```python
from build123d import *

# Parameters (mm, degrees)
BOSS_EXTRUDE1_DEPTH = 25.4
SKETCH2_R           = 9.801448676
SKETCH2_R_2         = 7.071368029
BOSS_EXTRUDE2_DEPTH = 19
BOSS_EXTRUDE3_DEPTH = 3.175
SKETCH4_R           = 3.175
CUT_EXTRUDE1_DEPTH  = 3.175


with BuildPart() as part:
    # Sketch1 → Boss-Extrude1 (new body)
    with BuildSketch(Plane.XY):
        Polygon((-76.495819173, -3.422180745), (-20.941461675, -3.422180745), (-1.20885062, 35.305249012), (-7.464460479, 16.03438497), (-18.995819173, -6.597180745), (-76.495819173, -6.597180745), align=None)
    extrude(amount=BOSS_EXTRUDE1_DEPTH)

    # Sketch2 → Boss-Extrude2 (add)
    with BuildSketch(Plane(origin=(0, -3.422180745, 0), x_dir=(1, 0, 0), z_dir=(0, 1, 0))):
        with Locations((-76.495819173, -12.7)):
            Circle(SKETCH2_R)
        with Locations((-76.495819173, -12.7)):
            Circle(SKETCH2_R_2, mode=Mode.SUBTRACT)
    extrude(amount=-BOSS_EXTRUDE2_DEPTH)

    # Sketch3 → Boss-Extrude3 (add)
    with BuildSketch(Plane(origin=(0, -3.422180745, 0), x_dir=(1, 0, 0), z_dir=(0, 1, 0))):
        Polygon((-76.495819173, -25.4), (-76.495819173, 0), (-85.929582176, -10.040580563), (-85.929582176, -15.359419437), align=None)
        Polygon((-85.929582176, -15.359419437), (-85.929582176, -10.040580563), (-86.297267848, -12.7), align=None)
    extrude(amount=-BOSS_EXTRUDE3_DEPTH)

    # Sketch4 → Cut-Extrude1 (cut)
    with BuildSketch(Plane(origin=(-15.240970814, 7.765662505, 0), x_dir=(0, 0, 1), z_dir=(-0.891006524, 0.4539905, 0))):
        with Locations((12.7, 18.20840051)):
            Circle(SKETCH4_R)
    extrude(amount=-CUT_EXTRUDE1_DEPTH, mode=Mode.SUBTRACT)


solid = part.part
```
Check sheet for the modelled part. Datum: model origin and axes. Units: mm. A direction names the side the tool comes from. Give positions to 0.01 mm unless a question says otherwise; leave off trailing zeros. Write each loop counter-clockwise with the first axis right and the second up, starting at its lowest first coordinate (ties: lowest second). Pieces come first, ordered by that corner, then holes. Notation, with made-up numbers: (6, 79) - (39, 79) arc R18 cw to (39, 102) - close; hole circle Ø9 at (71.5, 75). An arc over 180 degrees is marked (long way). Answer as a JSON object with one key per item and string values. Group by question number.
1) Access from +Z, -Z, +X, -X, +Y, -Y to the whole of each face (thin tool, end or side, straight path). Record for faces 4 (the face through (-76, -6.597, 13)), 5 (the face through (-78.094, -4.987, 1.701)), 6 (the face through (-54, -3.422, 13)).
2) Sectioned sample at D-D (z = 16.75). Record the cut outline in (x, y), then the cut area to 3 significant figures.
3) Release check for a two-part mould opening along Z. For faces 1 (the face through (-36, -4, 0)), 2 (the face through (-7.49, 20.773, 12.012)), 3 (the face through (-86.288, -14.9, 12.269)) record: pulls with the +Z half, pulls with the -Z half, needs draft (parallel to the pull), parting line crosses it, or undercut.
4) Sectioned sample at A-A (z = 12.7). Record the cut outline in (x, y), then the cut area to 3 significant figures.
5) Sectioned sample at B-B (x = -24.5). Record the cut outline in (y, z), then the cut area to 3 significant figures.
6) Thickness scan on probe 1 along X at (y, z) = (-12, 12.7); probe 2 along Y at (x, z) = (-59.5, 17.5); probe 3 along X at (y, z) = (-18.5, 17.75). Record the ranges inside material, lowest first. Write a range as from..to.
7) Depth check by flat-ended pin: P1, Ø8, axis at x = -76, z = 12.5, coming from the +Y side; P2, Ø10, axis at x = -11.5, z = 6, coming from the +Y side; P3, Ø5, axis at y = -12, z = 9, coming from the -X side. Enter the tip coordinate at first touch or a pass-through.
8) Sectioned sample at C-C (z = 23.5). Record the cut outline in (x, y), then the cut area to 3 significant figures.
Geometry results:
{
 "1": {"face 4": "-Y", "face 5": "-Z, -X, +Y, -Y", "face 6": "+Z, -Z, -X, +Y"},
 "2": {"outline": "(-85.42, -22.42) - (-82.29, -22.42) - (-82.29, -6.6) - (-70.7, -6.6) - (-70.7, -22.42) - (-67.57, -22.42) - (-67.57, -6.6) - (-19, -6.6) - (-7.46, 16.03) - (-1.21, 35.31) - (-20.94, -3.42) - (-85.42, -3.42) - close", "area": "416 mm^2"},
 "3": {"face 1": "pulls with the -Z half", "face 2": "undercut", "face 3": "parting line crosses it"},
 "4": {"outline": "(-86.3, -22.42) - (-83.57, -22.42) - (-83.57, -6.6) - (-69.42, -6.6) - (-69.42, -22.42) - (-66.69, -22.42) - (-66.69, -6.6) - (-19, -6.6) - (-7.46, 16.03) - (-6.17, 20.02) - (-8.42, 21.16) - (-20.94, -3.42) - (-86.3, -3.42) - close; (-5.53, 26.82) - (-4.19, 26.13) - (-1.21, 35.31) - close", "area": "394 mm^2"},
 "5": {"outline": "(-6.6, 0) - (-3.42, 0) - (-3.42, 25.4) - (-6.6, 25.4) - close", "area": "80.6 mm^2"},
 "6": {"probe 1": "x = -86.3..-83.57, -69.42..-66.69", "probe 2": "y = -6.6..-3.42", "probe 3": "x = -84.9..-81.45, -71.55..-68.1"},
 "7": {"P1": "stops at y = -3.42", "P2": "stops at y = 24.92", "P3": "stops at x = -86.22"},
 "8": {"outline": "(-78.28, -6.6) - (-19, -6.6) - (-7.46, 16.03) - (-1.21, 35.31) - (-20.94, -3.42) - (-78.28, -3.42) - close", "area": "294 mm^2"}
}
